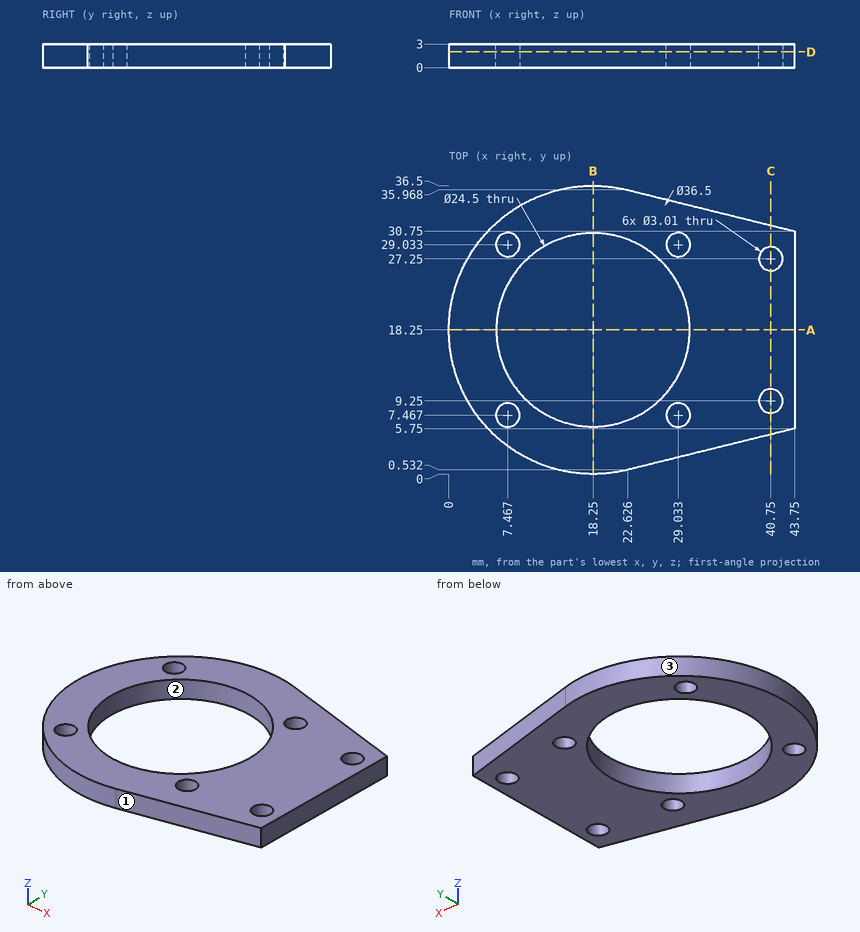
The drawing under review shows one solid part. Ordinate dimensions are in mm from its lowest x, y, z. Coordinates: 2 decimals unless noted, no trailing zeros. Order: outer loops, then holes, each group sorted by start corner. A loop starts at its lowest first (then second) coordinate and runs counter-clockwise, first axis right, second up. Notation, with made-up numbers: (87.25, 72) -> (100.25, 72) arc R11 ccw to (100.25, 87) -> close; hole circle Ø9 at (-37.5, -0.5). An arc over 180 degrees is marked (long way). Answer in a Markdown table with one row per item.
(1) The part is to be moulded in two halves that separate along X. For the marked faces 1, 2 and 3, say which applies: +X half, -X half, draft (parallel to the pull), parting line (faces both ways), or undercut.
Answers:
| item | result |
|---|---|
| face 1 | +X half |
| face 2 | undercut |
| face 3 | parting line |
(2) Consider section D-D (z = 2). State how many separate pieces and enclosed holes the cut face has.
Answers:
| item | result |
|---|---|
| separate pieces | 1 |
| enclosed holes | 7 |
(3) Consider section C-C (x = 40.75). Write out the cut boundary in (y, z) (1 decimal).
Answers:
| item | result |
|---|---|
| outline | (5, 0) -> (7.7, 0) -> (7.7, 3) -> (5, 3) -> close; (10.8, 0) -> (25.7, 0) -> (25.7, 3) -> (10.8, 3) -> close; (28.8, 0) -> (31.5, 0) -> (31.5, 3) -> (28.8, 3) -> close |
(4) Wall thickness on line 1 along Y through (x, z) = (28, 1.25) (1 decimal); line 2 along Y through (x, z) = (40.75, 1.1) (1 decimal); line 3 along Y through (x, z) = (9.5, 2.45) (1 decimal): over which ranges is each line inside the solid? List them lowest first.
Answers:
| item | result |
|---|---|
| line 1 | 1.9 to 6.4, 8.6 to 10.8, 25.7 to 27.9, 30.1 to 34.6 |
| line 2 | 5 to 7.7, 10.8 to 25.7, 28.8 to 31.5 |
| line 3 | 2.2 to 9.7, 26.8 to 34.3 |
(5) Consider section B-B (x = 18.25). Write out the cut boundary in (y, z), plus the area to 3 significant figures.
Answers:
| item | result |
|---|---|
| outline | (0, 0) -> (6, 0) -> (6, 3) -> (0, 3) -> close; (30.5, 0) -> (36.5, 0) -> (36.5, 3) -> (30.5, 3) -> close |
| area | 36.0 mm² |
(6) Consider section A-A (y = 18.25). Write out the cut boundary in (x, z).
Answers:
| item | result |
|---|---|
| outline | (0, 0) -> (6, 0) -> (6, 3) -> (0, 3) -> close; (30.5, 0) -> (43.75, 0) -> (43.75, 3) -> (30.5, 3) -> close |
(7) Insertion check: pin 1 (2.5 mm diameter, centred on x = 40.75, y = 27.25, fed in from -Z). The pin has a flat end and moves straight along its axis. Give the tip position at first contact, or say it passes through.
Answers:
| item | result |
|---|---|
| pin 1 | through |
